Autodesk Inventor part; units mm, degrees
ref_plane "YZ Plane" through (0, 0, 0) normal (1, 0, 0) x (0, 1, 0)
ref_plane "XZ Plane" through (0, 0, 0) normal (0, 1, 0) x (-1, 0, 0)
ref_plane "XY Plane" through (0, 0, 0) normal (0, 0, 1) x (1, 0, 0)
sketch "Sketch1" plane through (0, 0, 0) normal (0, 0, 1) x (1, 0, 0)
  line L0 (37.5, -25) -> (-37.5, -25)
  line L1 (-37.5, -25) -> (-37.5, 25)
  line L2 (-37.5, 25) -> (37.5, 25)
  line L3 (37.5, 25) -> (37.5, -25)
  line L4 (37.5, -25) -> (-37.5, 25) construction
  line L5 (-37.5, -25) -> (37.5, 25) construction
  point P0 (0, 0)
  dimension "d0" = 75
  dimension "d1" = 50
extrude "Extrusion1" add sketch "Sketch1" along normal blind 4
sketch "Sketch2" plane through (0, 0, 4) normal (0, 0, 1) x (1, 0, 0)
  point P0 (0, 0)
  point P1 (15.4, 10)
  point P2 (21, 0)
  point P3 (15.5, -10)
  point P4 (4.5, 10)
  point P5 (4.5, -10)
  point P6 (-1, 0)
hole "Hole1" at (15.4, 10, 4) at (21, 0, 4) at (15.5, -10, 4) at (4.5, 10, 4) at (4.5, -10, 4) at (-1, 0, 4) direction (0, 0, -1) diameter 10 end through all
sketch "Sketch3" plane through (0, 0, 4) normal (0, 0, 1) x (1, 0, 0)
  circle A0 centre (10, 0) radius 12.5
  line L0 (37.5, -25) -> (37.5, 25)
  point P0 (0, 0)
  dimension "d11" = 25
  dimension "d24" = 27.5
extrude "Extrusion2" cut sketch "Sketch3" against normal blind 10
sketch "Sketch4" plane through (0, 0, 4) normal (0, 0, 1) x (1, 0, 0)
  point P0 (0, 0)
  point P1 (30, 20)
  point P2 (30, -20)
  point P3 (-30, 20)
  point P4 (-30, -20)
hole "Hole2" at (30, 20, 4) at (30, -20, 4) at (-30, 20, 4) at (-30, -20, 4) direction (0, 0, -1) diameter 4.6 end through all
chamfer "Chamfer1" distance 2 angle 45 4 edges at (-30, -17.7, 4) (30, -17.7, 4) (-30, 22.3, 4) (30, 22.3, 4)
sketch "Sketch5" plane through (0, 0, 4) normal (0, 0, 1) x (1, 0, 0)
  point P0 (0, 0)
sketch "Sketch6" plane through (0, 0, 4) normal (0, 0, 1) x (1, 0, 0)
  line L0 (37.5, 25) -> (-37.5, 25)
  line L1 (-25, 25) -> (25, 25)
  line L2 (25, 25) -> (25, 22)
  line L3 (25, 22) -> (-25, 22)
  line L4 (-25, 22) -> (-25, 25)
  line L5 (-37.5, -25) -> (37.5, -25)
  line L6 (-25, -25) -> (25, -25)
  line L7 (25, -25) -> (25, -22)
  line L8 (25, -22) -> (-25, -22)
  line L9 (-25, -22) -> (-25, -25)
  point P0 (0, 0)
  dimension "d25" = 50
  dimension "d26" = 3
  dimension "d27" = 3
extrude "Extrusion3" add sketch "Sketch6" along normal blind 1
sketch "Sketch7" plane through (0, 0, 5) normal (0, 0, 1) x (1, 0, 0)
  line L0 (-25, 25) -> (-25, 22)
  line L1 (-25, 25) -> (25, 25)
  line L2 (25, 25) -> (25, 17.5)
  line L3 (25, 17.5) -> (-25, 17.5)
  line L4 (-25, 17.5) -> (-25, 25)
  line L5 (-37.5, -25) -> (37.5, -25)
  line L6 (-25, -25) -> (25, -25)
  line L7 (25, -25) -> (25, -17.5)
  line L8 (25, -17.5) -> (-25, -17.5)
  line L9 (-25, -17.5) -> (-25, -25)
  point P0 (0, 0)
  dimension "d30" = 50
  dimension "d31" = 7.5
  dimension "d32" = 7.5
extrude "Extrusion4" add sketch "Sketch7" along normal blind 3
properties part number "lid support"
Geometry: final body of the model. Coordinates: model frame, mm. A direction names the side the tool comes from. Coordinates: 2 decimals unless noted, no trailing zeros. Order: outer loops, then holes, each group sorted by start corner. A loop starts at its lowest first (then second) coordinate and runs counter-clockwise, first axis right, second up.
(1) Section query C-C (x = 4.5). Return the cut outline in (y, z), plus the area to 3 significant figures.
(2) Access query for faces 1 (the face through (-0.78, -6.33, 2.03)), 2 (the face through (0, -17.5, 6)), 3 (the face through (-25, -21, 6)), 4 (the face through (25, -21, 6)). Directions: +Z, -Z, +X, -X, +Y, -Y. A direction counts if a zero-diameter tool reaches every point of the face in a straight line with its end or side. Return the directions, or none.
(3) First-contact query: pin 1 (3 mm diameter, centred on y = -21.5, z = 6, fed in from +X); pin 2 (2 mm diameter, centred on y = -23, z = 6, fed in from -X); pin 3 (6 mm diameter, centred on x = 30, y = 20, fed in from +Z). Flat tips, straight axial feed; report the tip coordinate or a pass-through.
(4) Section query A-A (y = -20). Return the cut outline in (x, z), plus the area to 3 significant figures.
(5) Draft query along Y for faces 5 (the face through (-29.119, 17.875, 0.986)), 6 (the face through (1, -25, 4)), 7 (the face through (25, 21, 6)). Return one class per face: pulls with the +Y half, pulls with the -Y half, needs draft (parallel to the pull), parting line crosses it, or undercut.
(6) Material intervals for probe 1 along Y at (x, z) = (30, 1.25); probe 2 along X at (y, z) = (20, 0.95); probe 3 along X at (y, z) = (17, 3.75), sorted ascending.
(7) Section query B-B (x = -30). Return the cut outline in (y, z), plus the area to 3 significant figures.
(8) Section query D-D (y = -10). Return the cut outline in (x, z), plus the area to 3 significant figures.
Solution:
1. outline: (-25, 0) - (-15, 0) - (-15, 4) - (-22, 4) - (-22, 5) - (-17.5, 5) - (-17.5, 8) - (-25, 8) - close; (15, 0) - (25, 0) - (25, 8) - (17.5, 8) - (17.5, 5) - (22, 5) - (22, 4) - (15, 4) - close
1. area: 131 mm2
2. face 1: +Z, -Z
2. face 2: +Z, +X, -X
2. face 3: +Z, -X, +Y, -Y
2. face 4: +Z, +X, +Y, -Y
3. pin 1: stops at x = 25
3. pin 2: stops at x = -25
3. pin 3: stops at z = 2.7
4. outline: (-37.5, 0) - (-32.3, 0) - (-32.3, 2) - (-34.3, 4) - (-37.5, 4) - close; (-27.7, 0) - (27.7, 0) - (27.7, 2) - (25.7, 4) - (-25.7, 4) - (-27.7, 2) - close; (-25, 5) - (25, 5) - (25, 8) - (-25, 8) - close; (32.3, 0) - (37.5, 0) - (37.5, 4) - (34.3, 4) - (32.3, 2) - close
4. area: 405 mm2
5. face 5: undercut
5. face 6: pulls with the -Y half
5. face 7: needs draft
6. probe 1: y = -25 to -22.3, -17.7 to 17.7, 22.3 to 25
6. probe 2: x = -37.5 to -32.3, -27.7 to 27.7, 32.3 to 37.5
6. probe 3: x = -37.5 to -32.72, -27.28 to 27.28, 32.72 to 37.5
7. outline: (-25, 0) - (-22.3, 0) - (-22.3, 2) - (-24.3, 4) - (-25, 4) - close; (-17.7, 0) - (17.7, 0) - (17.7, 2) - (15.7, 4) - (-15.7, 4) - (-17.7, 2) - close; (22.3, 0) - (25, 0) - (25, 4) - (24.3, 4) - (22.3, 2) - close
7. area: 155 mm2
8. outline: (-37.5, 0) - (-0.5, 0) - (-0.5, 4) - (-37.5, 4) - close; (20.5, 0) - (37.5, 0) - (37.5, 4) - (20.5, 4) - close
8. area: 216 mm2
